```python
from build123d import *

# Parameters (mm, degrees)
F0_R     = 50.8
F2_DEPTH = 177.8
F3_R     = 38.1
F4_DEPTH = 177.801
F1_R     = 41.91
F7_DEPTH = 177.801


with BuildPart() as f2:
    # F0 (on Top) → F2 (new body)
    with BuildSketch(Plane.XY):
        Circle(F0_R)
    extrude(amount=F2_DEPTH)

    # F3 (on face) → F4 (cut, through all)
    with BuildSketch(Plane.XY.offset(177.8)):
        Circle(F3_R)
    extrude(amount=-F4_DEPTH, mode=Mode.SUBTRACT)

    # F5 (on Front) → F6 (revolve)
    with BuildSketch(Plane.XZ):
        with BuildLine():
            ThreePointArc((100.0125, 0), (70.9357679727, 13.9783849732), (49.5876034492, 38.167379647))
            Line((49.5876034492, 38.167379647), (49.5876034492, 0))
            Line((49.5876034492, 0), (100.0125, 0))
        make_face()
    revolve(axis=Axis((0, 0, 0), (0, 0, -1)))

    # F1 (on Top) → F7 (cut, through all)
    with BuildSketch(Plane.XY):
        with Locations((-92.71, 0)):
            Circle(F1_R)
        with Locations((-46.355, -80.2892151849)):
            Circle(F1_R)
        with Locations((46.355, -80.2892151849)):
            Circle(F1_R)
        with Locations((92.71, 0)):
            Circle(F1_R)
        with Locations((46.355, 80.2892151849)):
            Circle(F1_R)
        with Locations((-46.355, 80.2892151849)):
            Circle(F1_R)
    extrude(amount=F7_DEPTH, mode=Mode.SUBTRACT)

    # F8 (on Front) → F9 (revolve, cut)
    with BuildSketch(Plane.XZ):
        with BuildLine():
            Line((-50.8, 177.8), (-50.8, 36.134957756))
            ThreePointArc((-50.8, 36.134957756), (-45.1399977249, 46.3755737202), (-43.18, 57.9109215693))
            Line((-43.18, 57.9109215693), (-43.18, 177.8))
            Line((-43.18, 177.8), (-50.8, 177.8))
        make_face()
    revolve(axis=Axis((0, 0, 177.8), (0, 0, -1)), mode=Mode.SUBTRACT)


solid = f2.part
```
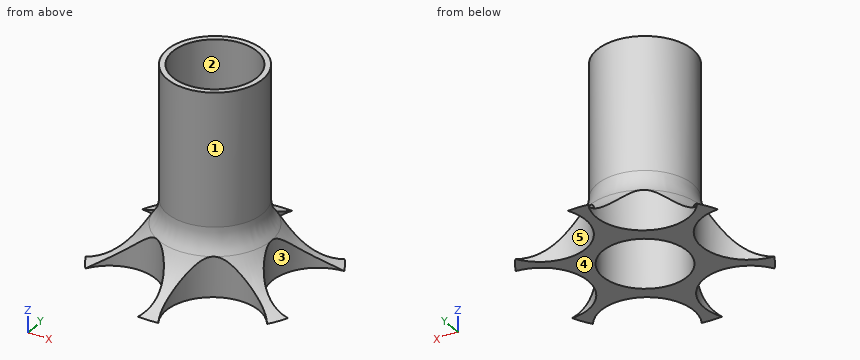
The model under review builds one solid part; all positions refer to its coordinate system, in mm. Face numbers are marked on the shaded views. A direction names the side the tool comes from. Give positions to 0.01 mm unless a question says otherwise; leave off trailing zeros. Write each loop counter-clockwise with the first axis right and the second up, starting at its lowest first coordinate (ties: lowest second). Pieces come first, ordered by that corner, then holes.
(1) Tool access review of the marked faces 1 and 2: name each direction out of +Z, -Z, +X, -X, +Y, -Y from which nothing blocks a thin tool from reaching the whole face with its end or side.
(2) Consider section B-B, the plane z = 123. Give the boundary of the cut face in (x, y).
(3) The part is to be moulded in two halves that separate along X. For the marked faces 3, 4 and 5, say which applies: released by +X, released by -X, zero draft, split by the parting line, or undercut.
(4) To check wall thickness, follow L1, parallel to Y at x = 0, z = 73; L2, parallel to Y at x = 0, z = 39; L3, parallel to X at y = -14, z = 17.5. State the ranges of each line that lie inside material, in increasing order.
(5) For P1, Ø12, axis at y = -3, z = 22, coming from the +X side; P2, Ø6, axis at y = -31.5, z = 148, coming from the +X side; P3, Ø6, axis at x = 0.5, z = 120.5, coming from the -Y side, all flat-tipped, find the tip position at first contact; note any pin that passes through.
Returned:
1. face 1: +Z
1. face 2: +Z, -Z
2. outline: circle Ø86.36 at (0, 0); hole circle Ø76.2 at (0, 0)
3. face 3: released by +X
3. face 4: zero draft
3. face 5: undercut
4. L1: y = -43.18 to -38.1, 38.1 to 43.18
4. L2: y = -48.74 to -38.1, 38.1 to 48.74
4. L3: x = -53.21 to -35.43, 35.43 to 53.21
5. P1: stops at x = 51.78
5. P2: stops at x = 32.44
5. P3: stops at y = -43.18
